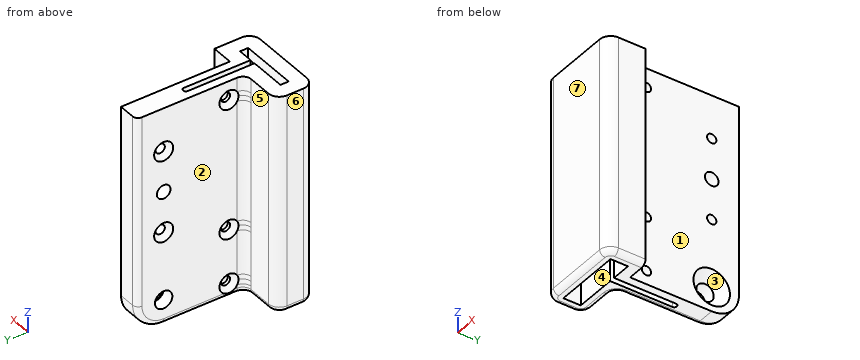
from build123d import *

# Parameters (mm, degrees)
PAD_DEPTH       = 80
POCKET_DEPTH    = 76
SKETCH002_R     = 1.7
SKETCH002_R_2   = 3.2
SKETCH002_R_3   = 2.5
POCKET001_DEPTH = 16.001
POCKET002_DEPTH = 5
CHAMFER_SIZE    = 3.5
FILLET_R        = 10
CHAMFER001_SIZE = 1.8
CHAMFER002_SIZE = 1.8
CHAMFER003_SIZE = 1.8
CHAMFER004_SIZE = 1.8
CHAMFER005_SIZE = 1.8
FILLET001_R     = 3
FILLET002_R     = 4
FILLET003_R     = 4
FILLET004_R     = 4
FILLET005_R     = 2
FILLET006_R     = 0.9
FILLET007_R     = 0.9


with BuildPart() as fillet007:
    # Sketch → Pad (new body)
    with BuildSketch(Plane.XY):
        Polygon((-4, 0), (-4, 40), (4, 40), (4, 18), (4, 0), (12, 0), (12, -14), (-20, -14), (-20, 0), align=None)
    extrude(amount=PAD_DEPTH)

    # Sketch001 → Pocket (cut)
    with BuildSketch(Plane.XY.offset(80)):
        Polygon((1, -3.8), (1, 20), (-1, 20), (-1, -3.8), (-16.25, -3.8), (-16.25, -10.2), (8.25, -10.2), (8.25, -3.8), align=None)
    extrude(amount=-POCKET_DEPTH, mode=Mode.SUBTRACT)

    # Sketch002 → Pocket001 (cut, through all)
    with BuildSketch(Plane(origin=(-4, 0, 0), x_dir=(0, -1, 0), z_dir=(-1, 0, 0))):
        with Locations((-6, 7)):
            Circle(SKETCH002_R)
        with Locations((-6, 55)):
            Circle(SKETCH002_R)
        with Locations((-6, 75)):
            Circle(SKETCH002_R)
        with Locations((-30, 46)):
            Circle(SKETCH002_R)
        with Locations((-30, 16)):
            Circle(SKETCH002_R)
        with Locations((-30, 71)):
            Circle(SKETCH002_R_2)
        with Locations((-30, 31)):
            Circle(SKETCH002_R_3)
    extrude(amount=-POCKET001_DEPTH, mode=Mode.SUBTRACT)

    # Sketch003 → Pocket002 (cut)
    with BuildSketch(Plane(origin=(0, 0, 0), x_dir=(1, 0, 0), z_dir=(0, 0, -1))):
        Polygon((-14.5, 8.5), (6.5, 8.5), (6.5, 5.5), (1, 5.5), (1, -20), (-1, -20), (-1, 5.5), (-14.5, 5.5), align=None)
    extrude(amount=-POCKET002_DEPTH, mode=Mode.SUBTRACT)

    # Chamfer
    chamfer_edges = [fillet007.edges().sort_by_distance(p)[0] for p in [
        (4, 33.2, 71),
    ]]
    chamfer(chamfer_edges, length=CHAMFER_SIZE)

    # Fillet
    fillet_edges = [fillet007.edges().sort_by_distance(p)[0] for p in [
        (0, 40, 80),
    ]]
    fillet(fillet_edges, radius=FILLET_R)

    # Chamfer001
    chamfer001_edges = [fillet007.edges().sort_by_distance(p)[0] for p in [
        (-4, 7.7, 7),
    ]]
    chamfer(chamfer001_edges, length=CHAMFER001_SIZE)

    # Chamfer002
    chamfer002_edges = [fillet007.edges().sort_by_distance(p)[0] for p in [
        (-4, 7.7, 75),
    ]]
    chamfer(chamfer002_edges, length=CHAMFER002_SIZE)

    # Chamfer003
    chamfer003_edges = [fillet007.edges().sort_by_distance(p)[0] for p in [
        (-4, 7.7, 55),
    ]]
    chamfer(chamfer003_edges, length=CHAMFER003_SIZE)

    # Chamfer004
    chamfer004_edges = [fillet007.edges().sort_by_distance(p)[0] for p in [
        (-4, 31.7, 46),
    ]]
    chamfer(chamfer004_edges, length=CHAMFER004_SIZE)

    # Chamfer005
    chamfer005_edges = [fillet007.edges().sort_by_distance(p)[0] for p in [
        (-4, 31.7, 16),
    ]]
    chamfer(chamfer005_edges, length=CHAMFER005_SIZE)

    # Fillet001
    fillet001_edges = [fillet007.edges().sort_by_distance(p)[0] for p in [
        (-4, 0, 40),
    ]]
    fillet(fillet001_edges, radius=FILLET001_R)

    # Fillet002
    fillet002_edges = [fillet007.edges().sort_by_distance(p)[0] for p in [
        (-20, 0, 40),
    ]]
    fillet(fillet002_edges, radius=FILLET002_R)

    # Fillet003
    fillet003_edges = [fillet007.edges().sort_by_distance(p)[0] for p in [
        (-20, -14, 40),
    ]]
    fillet(fillet003_edges, radius=FILLET003_R)

    # Fillet004
    fillet004_edges = [fillet007.edges().sort_by_distance(p)[0] for p in [
        (12, -14, 40),
    ]]
    fillet(fillet004_edges, radius=FILLET004_R)

    # Fillet005
    fillet005_edges = [fillet007.edges().sort_by_distance(p)[0] for p in [
        (-4, 40, 35),
    ]]
    fillet(fillet005_edges, radius=FILLET005_R)

    # Fillet006
    fillet006_edges = [fillet007.edges().sort_by_distance(p)[0] for p in [
        (-1, 20, 40),
    ]]
    fillet(fillet006_edges, radius=FILLET006_R)

    # Fillet007
    fillet007_edges = [fillet007.edges().sort_by_distance(p)[0] for p in [
        (1, 20, 40),
    ]]
    fillet(fillet007_edges, radius=FILLET007_R)


with BuildPart() as part_mirroring:
    # Part__Mirroring: instance of Fillet007
    add(fillet007.part.mirror(Plane(origin=(0, 0, 0), x_dir=(0, 1, 0), z_dir=(0, 0, 1))))


solid = part_mirroring.part
The listing builds one solid part. Answer for the finished solid, in the listing's coordinates (mm). Face numbers are marked on the shaded views. A direction names the side the tool comes from. Coordinates: 2 decimals unless noted, no trailing zeros. Loops run counter-clockwise (first coordinate to the right, second up) from the corner with the lowest first, then second, coordinate; pieces in that order, holes last.
1) Find section C-C on z = -36.5. Write down the section's boundary in (x, y).
2) Find section B-B on x = -11. Write down the section's boundary in (y, z).
3) Flat-ended cylindrical pins translate along their axes: pin 1 Ø1.3 at (y, z) = (3.5, -77.5) entering from -X; pin 2 Ø3 at (x, z) = (-6, -18.5) entering from +Y; pin 3 Ø2.5 at (y, z) = (30, -46) entering from -X; pin 4 Ø7.5 at (x, z) = (-6.5, -30) entering from +Y. Find the tip coordinate at first contact, or state that the pin passes through.
4) Determine the mould class of the marked faces 4, 5, 6 and 7 for opening direction Y: pulls with the +Y half, pulls with the -Y half, needs draft (parallel to the pull), parting line crosses it, or undercut.
5) A tool of negligible diameter and unlimited length cuts with its end or side. For the marked faces 1, 2 and 3, from which of +Z, -Z, +X, -X, +Y, -Y can it reach the whole face along a straight path? Write none if from no direction.
6) Find the intervals of material crossed by L1, parallel to Y at x = -0.25, z = -46; L2, parallel to Y at x = 3.2, z = -7; L3, parallel to Z at x = 0, y = 30, in increasing order.
7) Find section A-A on z = -46. Give the number of separate pieces and of enclosed holes in the cut face, then the cut area to 3 significant figures.
Values:
1. outline: (-20, -10) arc R4 ccw to (-16, -14) - (8, -14) arc R4 ccw to (12, -10) - (12, 0) - (4, 0) - (4, 40) - (-2, 40) arc R2 ccw to (-4, 38) - (-4, 3) arc R3 cw to (-7, 0) - (-16, 0) arc R4 ccw to (-20, -4) - close; hole (-16.25, -10.2) - (8.25, -10.2) - (8.25, -3.8) - (1, -3.8) - (1, 19.1) arc R0.9 ccw to (0.1, 20) - (-0.1, 20) arc R0.9 ccw to (-1, 19.1) - (-1, -3.8) - (-16.25, -3.8) - close
2. outline: (-14, -78) arc R2 ccw to (-12, -80) - (-10.2, -80) - (-10.2, -4) - (-8.5, -4) - (-8.5, 0) - (-14, 0) - close; (-5.5, -4) - (-3.8, -4) - (-3.8, -80) - (-2, -80) arc R2 ccw to (0, -78) - (0, 0) - (-5.5, 0) - close
3. pin 1: stops at x = -4
3. pin 2: stops at y = 1.34
3. pin 3: passes through
3. pin 4: stops at y = 39.85
4. face 4: undercut
4. face 5: pulls with the +Y half
4. face 6: needs draft
4. face 7: pulls with the -Y half
5. face 1: +Z, -Z, +X, +Y
5. face 2: +Z, -Z, -X, +Y
5. face 3: +X
6. L1: y = -14 to -10.2, 19.99 to 28.3, 31.7 to 40
6. L2: y = -14 to -10.2, -3.8 to 4.3, 7.7 to 40
6. L3: z = -80 to -74.2, -67.8 to -47.7, -44.3 to -33.5, -28.5 to -17.7, -14.3 to 0
7. separate pieces: 2
7. enclosed holes: 1
7. area: 524 mm2
